from build123d import *

# Parameters (mm, degrees)
SKETCH1_W           = 650
SKETCH1_H           = 170
BOSS_EXTRUDE1_DEPTH = 482
SKETCH2_R           = 16
CUT_EXTRUDE1_DEPTH  = 483
SKETCH3_W           = 630
SKETCH3_H           = 462
CUT_EXTRUDE2_DEPTH  = 150


with BuildPart() as part:
    # Sketch1 → Boss-Extrude1 (new body)
    with BuildSketch(Plane.XY):
        Rectangle(SKETCH1_W, SKETCH1_H)
    extrude(amount=BOSS_EXTRUDE1_DEPTH)

    # Sketch2 → Cut-Extrude1 (cut, through all)
    with BuildSketch(Plane(origin=(0, 0, 0), x_dir=(-1, 0, 0), z_dir=(0, 0, -1))):
        with Locations((0, 15)):
            Circle(SKETCH2_R)
    extrude(amount=-CUT_EXTRUDE1_DEPTH, mode=Mode.SUBTRACT)

    # Sketch3 → Cut-Extrude2 (cut)
    with BuildSketch(Plane(origin=(0, 85, 0), x_dir=(1, 0, 0), z_dir=(0, 1, 0))):
        with Locations((0, -241)):
            Rectangle(SKETCH3_W, SKETCH3_H)
    extrude(amount=-CUT_EXTRUDE2_DEPTH, mode=Mode.SUBTRACT)


solid = part.part
Geometry: final body of the model. Coordinates: model frame, mm. A direction names the side the tool comes from. Round coordinates to 2 decimals unless told otherwise and drop trailing zeros. Order: outer loops, then holes, each group sorted by start corner. A loop starts at its lowest first (then second) coordinate and runs counter-clockwise, first axis right, second up.
Q1. Pin query (flat end, axial travel): pin 1 (4 mm diameter, centred on x = 165, z = 122.5, fed in from +Y); pin 2 (1.5 mm diameter, centred on x = -7, y = 2.5, fed in from -Z). Return the tip coordinate at first contact, or that it passes through.
Result sheet:
pin 1: stops at y = -65
pin 2: passes through
Q2. Mould query, pull axis X, two halves, no side actions, for faces 3 (the face through (3.47, -0.62, 4.93)), 4 (the face through (-4, -6, 10)), 5 (the face through (-325, -1, 238)), 6 (the face through (-2, 85, 8)). Classes: released by +X, released by -X, zero draft, split by the parting line, or undercut.
Result sheet:
face 3: undercut
face 4: undercut
face 5: released by -X
face 6: zero draft
Q3. Material intervals for probe 1 along Y at (x, z) = (0, 479.5); probe 2 along X at (y, z) = (76.5, 440); probe 3 along Z at (x, y) = (143, 38.5), sorted ascending.
Result sheet:
probe 1: y = -85 to -1, 31 to 85
probe 2: x = -325 to -315, 315 to 325
probe 3: z = 0 to 10, 472 to 482
Q4. Section B-B, the plane y = 15. Output: boundary loops of the cut face in (x, z), and give its area (3 significant figures).
Result sheet:
outline: (-325, 0) - (-16, 0) - (-16, 10) - (-315, 10) - (-315, 472) - (-16, 472) - (-16, 482) - (-325, 482) - close; (16, 0) - (325, 0) - (325, 482) - (16, 482) - (16, 472) - (315, 472) - (315, 10) - (16, 10) - close
area: 21,600 mm2
Q5. Access query for faces 1 (the face through (-315, 11, 244)), 2 (the face through (-5, -85, 238)). Directions: +Z, -Z, +X, -X, +Y, -Y. A direction counts if a zero-diameter tool reaches every point of the face in a straight line with its end or side. Return the directions, or none.
Result sheet:
face 1: +Y
face 2: +Z, -Z, +X, -X, -Y
Q6. Section C-C, the plane y = -55. Output: boundary loops of the cut face in (x, z), and give its area (3 significant figures).
Result sheet:
outline: (-325, 0) - (325, 0) - (325, 482) - (-325, 482) - close; hole (-315, 10) - (315, 10) - (315, 472) - (-315, 472) - close
area: 22,200 mm2
Q7. Section A-A, the plane x = 0. Output: boundary loops of the cut face in (y, z), and give its area (3 significant figures).
Result sheet:
outline: (-85, 0) - (-1, 0) - (-1, 10) - (-65, 10) - (-65, 472) - (-1, 472) - (-1, 482) - (-85, 482) - close; (31, 0) - (85, 0) - (85, 10) - (31, 10) - close; (31, 472) - (85, 472) - (85, 482) - (31, 482) - close
area: 12,000 mm2
Q8. Section D-D, the plane x = 141. Output: boundary loops of the cut face in (y, z), and give its area (3 significant figures).
Result sheet:
outline: (-85, 0) - (85, 0) - (85, 10) - (-65, 10) - (-65, 472) - (85, 472) - (85, 482) - (-85, 482) - close
area: 12,600 mm2
